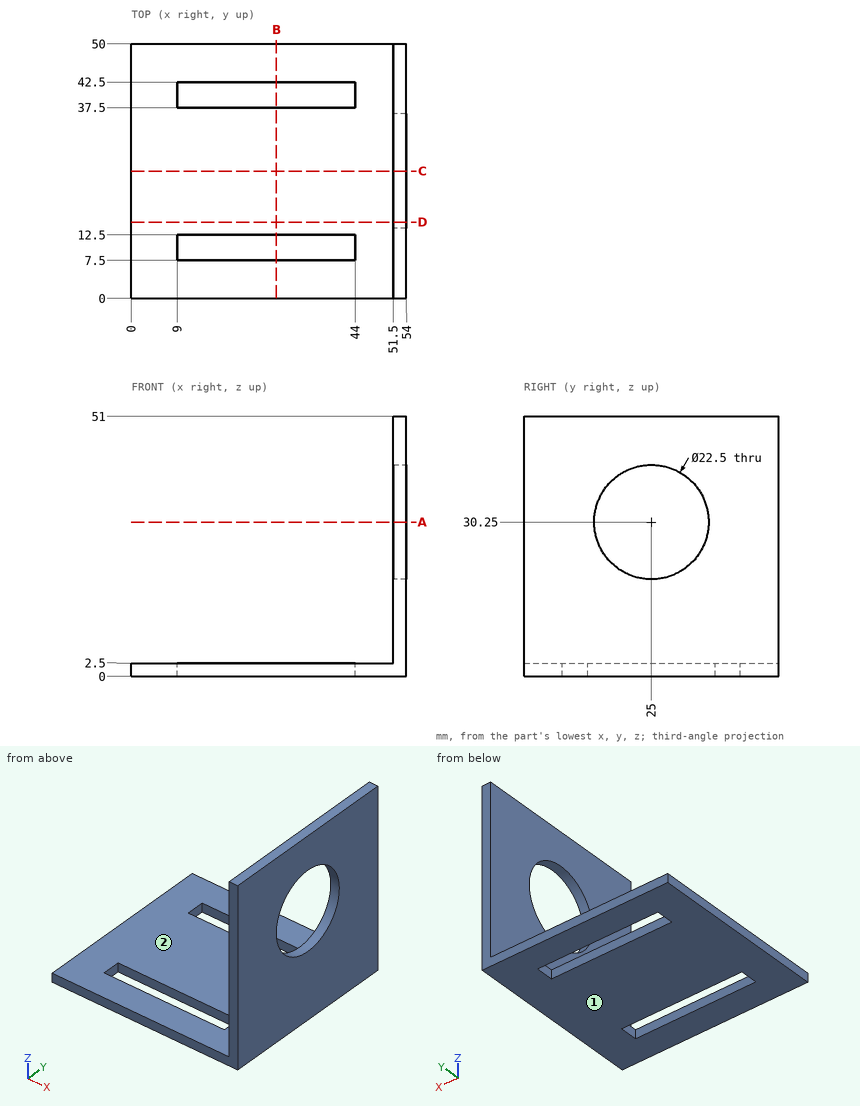
Input: dimensioned drawing with shaded views. Units: mm. Origin: part minimum x, y, z. A direction names the side the tool comes from. Round coordinates to 2 decimals unless told otherwise and drop trailing zeros. Order: outer loops, then holes, each group sorted by start corner. A loop starts at its lowest first (then second) coordinate and runs counter-clockwise, first axis right, second up. Notation, with made-up numbers: (82, 33.5) - (127, 33.5) arc R21 ccw to (127, 68.5) - close; hole circle Ø4 at (32, -4). An arc over 180 degrees is marked (long way). Write item = value, one per line. Start each with the question number.
Q1. Cut plane B-B on x = 28.5. Return the cut outline in (y, z), and give its area (3 significant figures).
Q2. Pin query (flat end, axial travel): pin 1 (5 mm diameter, centred on x = 20.5, y = 7.5, fed in from +Z); pin 2 (1 mm diameter, centred on y = 30.5, z = 11, fed in from -X). Return the tip coordinate at first contact, or that it passes through.
Q3. Cut plane D-D on y = 15. Return the cut outline in (x, z).
Q4. Access query for the marked faces 1 and 2. Directions: +Z, -Z, +X, -X, +Y, -Y. A direction counts if a zero-diameter tool reaches every point of the face in a straight line with its end or side. Return the directions, or none.
Q5. Cut plane C-C on y = 25. Return the cut outline in (x, z), and give its area (3 significant figures).
Q6. Cut plane A-A on z = 30.25. Return the cut outline in (x, y), and give its area (4 significant figures).
Q7. Ray query, line 1 (Y direction, x = 52.95, z = 30.25); line 2 (Z direction, x = 9.5, y = 28); line 3 (X direction, y = 21, z = 7). Return the intervals inside material, ascending. Write a range as from..to.
Outcome:
q1.outline = (0, 0) - (7.5, 0) - (7.5, 2.5) - (0, 2.5) - close; (12.5, 0) - (37.5, 0) - (37.5, 2.5) - (12.5, 2.5) - close; (42.5, 0) - (50, 0) - (50, 2.5) - (42.5, 2.5) - close
q1.area = 100 mm^2
q2.pin_1 = 2.5
q2.pin_2 = 51.5
q3.outline = (0, 0) - (54, 0) - (54, 25.1) - (51.5, 25.1) - (51.5, 2.5) - (0, 2.5) - close; (51.5, 35.4) - (54, 35.4) - (54, 51) - (51.5, 51) - close
q4.face_1 = -Z, +X, -X, +Y, -Y
q4.face_2 = +Z, -X, +Y, -Y
q5.outline = (0, 0) - (54, 0) - (54, 19) - (51.5, 19) - (51.5, 2.5) - (0, 2.5) - close; (51.5, 41.5) - (54, 41.5) - (54, 51) - (51.5, 51) - close
q5.area = 200 mm^2
q6.outline = (51.5, 0) - (54, 0) - (54, 13.75) - (51.5, 13.75) - close; (51.5, 36.25) - (54, 36.25) - (54, 50) - (51.5, 50) - close
q6.area = 68.75 mm^2
q7.line_1 = 0..13.75, 36.25..50
q7.line_2 = 0..2.5
q7.line_3 = 51.5..54
